Part print with two shaded views. Sizes in mm from the minimum x, y, z corner. A direction names the side the tool comes from. Give positions to 0.01 mm unless a question says otherwise; leave off trailing zeros. Order: outer loops, then holes, each group sorted by start corner. A loop starts at its lowest first (then second) coordinate and runs counter-clockwise, first axis right, second up. Notation, with made-up numbers: (56, 58) -> (85, 58) arc R33 cw to (85, 89) -> close; hole circle Ø10 at (38.5, 69.25). An arc over 180 degrees is marked (long way). Answer as CSV lines item,"result".
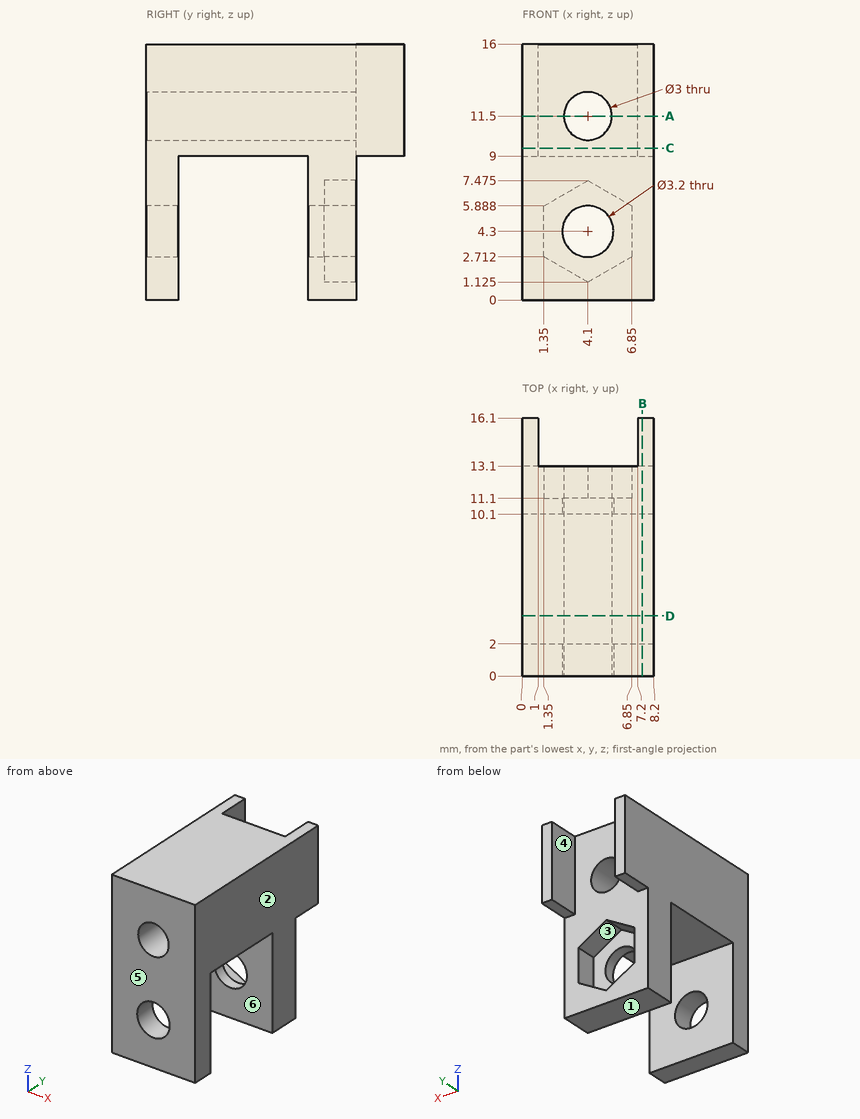
1) Band-saw the part on A-A, the plane z = 11.5. Write the cut outline in (x, y).
Data:
outline,"(0, 0) -> (2.6, 0) -> (2.6, 13.1) -> (1, 13.1) -> (1, 16.1) -> (0, 16.1) -> close; (5.6, 0) -> (8.2, 0) -> (8.2, 16.1) -> (7.2, 16.1) -> (7.2, 13.1) -> (5.6, 13.1) -> close"
2) Band-saw the part on B-B, the plane x = 7.5. Write the cut outline in (y, z).
Data:
outline,"(0, 0) -> (2, 0) -> (2, 9) -> (10.1, 9) -> (10.1, 0) -> (13.1, 0) -> (13.1, 9) -> (16.1, 9) -> (16.1, 16) -> (0, 16) -> close"
3) Band-saw the part on C-C, the plane z = 9.5. Write the cut outline in (x, y), then the cut area to 3 significant figures.
Data:
outline,"(0, 0) -> (8.2, 0) -> (8.2, 16.1) -> (7.2, 16.1) -> (7.2, 13.1) -> (1, 13.1) -> (1, 16.1) -> (0, 16.1) -> close"
area,"113 mm2"
4) Wall check: line 1 along Y through (x, z) = (1, 7.5); line 2 along X through (y, z) = (9, 11.5); line 3 along X through (y, z) = (1.5, 4.3). Give the ranges that are in metal, low to high. Write a range as [from, to].
Data:
line 1,"y = [0, 2], [10.1, 13.1]"
line 2,"x = [0, 2.6], [5.6, 8.2]"
line 3,"x = [0, 2.5], [5.7, 8.2]"
5) Band-saw the part on D-D, the plane y = 3.75. Write the cut outline in (x, z).
Data:
outline,"(0, 9) -> (8.2, 9) -> (8.2, 16) -> (0, 16) -> close; hole circle Ø3 at (4.1, 11.5)"
6) Pin check, flat tips, straight feed: P1, Ø1, axis at x = 5, y = 6, coming from the -Z side; P2, Ø3, axis at x = 4, z = 12.5, coming from the +Y side; P3, Ø3, axis at y = 4.5, z = 6.5, coming from the -X side; P4, Ø4, axis at x = 4.1, z = 4.3, coming from the +Y side. Stop position of each tip, or through.
Data:
P1,"stops at z = 9"
P2,"stops at y = 13.1"
P3,"passes through"
P4,"stops at y = 11.1"
7) Pull direction X, two halves, no side cores. Call the marked faces 1, 2 and 3: pulls with the +X half, pulls with the -X half, needs draft (parallel to the pull), parting line crosses it, or undercut.
Data:
face 1,"needs draft"
face 2,"pulls with the +X half"
face 3,"undercut"
8) Which spindle directions (+Z, -Z, +X, -X, +Y, -Y) get a long thin tool onto all of the face, cutting with end or side? Do the marked faces 4, 5 and 6. Say none if no direction does.
Data:
face 4,"+Z, -Z, +Y"
face 5,"+Z, -Z, +X, -X, -Y"
face 6,"-Z, +X, -X"
